Can you work these out from the model? Positions are in its coordinate system, mm. A direction names the side the tool comes from. Round coordinates to 2 decimals unless told otherwise and drop trailing zeros. Write each loop counter-clockwise with the first axis right and the second up, starting at its lowest first coordinate (ties: lowest second). Pieces come first, ordered by that corner, then holes. Notation, with made-up numbers: (-17, 21.25) -> (23, 21.25) arc R22 ccw to (23, 30.25) -> close; hole circle Ø10 at (-28.5, 31). An arc over 180 degrees is marked (long way). Write item = value, one per line. Start each with the question number.
1) If I drill on line 1 (Y direction, x = 0, z = 1.75); line 2 (Z direction, x = -7.5, y = 41.5); line 3 (X direction, y = 1, z = 1.5), over which ranges is the centre line in solid material (lowest first)?
2) Imagine slicing it at B-B, the plane y = 0. Please give me the cut outline in (x, z), then the cut area to 3 significant figures.
3) Imagine slicing it at D-D, the plane y = 16.5. Please give me the cut outline in (x, z), then the cut area to 3 significant figures.
4) I'm going to push flat-ended pins straight in: pin 1 (2.5 mm diameter, centred on x = -8.01, y = 37.25, fed in from -Z); pin 2 (2 mm diameter, centred on x = -2, y = 34, fed in from +Z); pin 3 (3 mm diameter, centred on x = -11, z = 1.5, fed in from +Y). Where does each tip first touch, or does it pass through?
5) Imagine slicing it at A-A, the plane x = 0. Please give me the cut outline in (y, z).
6) For faces 1 (the face through (-3.42, 3.13, 3.28)), 2 (the face through (-7.54, 36.35, 0.15)), which set-ups out of +Z, -Z, +X, -X, +Y, -Y let a thin tool reach every point of the face, with its end or its side?
7) Thinking about a two-plate mould opening in Y: for faces 3 (the face through (-10.27, 17.55, 0.78)), 4 (the face through (-2.217, -1.7, 3.131)), 5 (the face through (0, 43.598, 1)), 6 (the face through (7.793, 36.256, 0.15)), which applies, +Y half, -Y half, draft (parallel to the pull), parting line (faces both ways), or undercut?
8) Imagine slicing it at C-C, the plane z = 3.75. Please give me the cut outline in (x, y), then the cut area to 3 significant figures.
from build123d import *

# Parameters (mm, degrees)
F0_R     = 4.6355
F0_R_2   = 1.016
F1_DEPTH = 1.5748
F0_R_3   = 2.794
F2_DEPTH = 6.35
F3_SIZE  = 1.27


# Not quite as in the source:
# - a fillet or chamfer that OpenCascade refuses, or shapes differently, is made with other operations: its cross-section is extruded or revolved along the edge and cut away or added
# - a feature names something its author has since deleted; it is built from what else it names


with BuildPart() as f1:
    # F0 (on Top) → F1 (new body)
    with BuildSketch(Plane.XY):
        with BuildLine():
            Line((-14.2215059748, 35.912132599), (-6.2079540965, -1.3355919797))
            ThreePointArc((-6.2079540965, -1.3355919797), (0, -6.35), (6.2079540965, -1.3355919797))
            Line((6.2079540965, -1.3355919797), (14.2215059748, 35.912132599))
            ThreePointArc((14.2215059748, 35.912132599), (12.9533650869, 41.2378054632), (8.0135518783, 43.5977245787))
            Line((8.0135518783, 43.5977245787), (-8.0135518783, 43.5977245787))
            ThreePointArc((-8.0135518783, 43.5977245787), (-12.9533650869, 41.2378054632), (-14.2215059748, 35.912132599))
        make_face()
        Circle(F0_R, mode=Mode.SUBTRACT)
        with Locations((-8.0135518783, 37.2477245787)):
            Circle(F0_R_2, mode=Mode.SUBTRACT)
        with Locations((8.0135518783, 37.2477245787)):
            Circle(F0_R_2, mode=Mode.SUBTRACT)
    extrude(amount=F1_DEPTH)

    # F0 (on Top) → F2 (join)
    with BuildSketch(Plane.XY):
        Circle(F0_R)
        Circle(F0_R_3, mode=Mode.SUBTRACT)
    extrude(amount=F2_DEPTH)

    # F3
    f3_edges = [f1.edges().sort_by_distance(p)[0] for p in [
        (-9.029552, 37.247725, 1.5748),
        (6.997552, 37.247725, 1.5748),
    ]]
    chamfer(f3_edges, length=F3_SIZE)

    # F4: chamfer of 0.762 x 1.3198227154 on 1 edges, made by hand

    # F4_s1 → F4_t2 (revolve, cut)
    with BuildSketch(Plane.XZ):
        Polygon((4.6355, 5.0301772846), (3.8735, 6.35), (4.6355, 6.35), align=None)
    revolve(axis=Axis((0, 0, 6.35), (0, 0, 1)), mode=Mode.SUBTRACT)


solid = f1.part
Reported:
q1.line_1 = -4.64 to -2.79, 2.79 to 4.64
q1.line_2 = 0 to 1.57
q1.line_3 = -6.71 to -2.61, 2.61 to 6.71
q2.outline = (-6.5, 0) -> (-2.79, 0) -> (-2.79, 6.35) -> (-3.87, 6.35) -> (-4.64, 5.03) -> (-4.64, 1.57) -> (-6.5, 1.57) -> close; (2.79, 0) -> (6.5, 0) -> (6.5, 1.57) -> (4.64, 1.57) -> (4.64, 5.03) -> (3.87, 6.35) -> (2.79, 6.35) -> close
q2.area = 28.2 mm²
q3.outline = (-10.05, 0) -> (10.05, 0) -> (10.05, 1.57) -> (-10.05, 1.57) -> close
q3.area = 31.6 mm²
q4.pin_1 = 0
q4.pin_2 = 1.57
q4.pin_3 = 43.42
q5.outline = (-6.35, 0) -> (-2.79, 0) -> (-2.79, 6.35) -> (-3.87, 6.35) -> (-4.64, 5.03) -> (-4.64, 1.57) -> (-6.35, 1.57) -> close; (2.79, 0) -> (43.6, 0) -> (43.6, 1.57) -> (4.64, 1.57) -> (4.64, 5.03) -> (3.87, 6.35) -> (2.79, 6.35) -> close
q6.face_1 = +Z
q6.face_2 = +Z, -Z
q7.face_3 = -Y half
q7.face_4 = undercut
q7.face_5 = +Y half
q7.face_6 = undercut
q8.outline = circle Ø9.27 at (0, 0); hole circle Ø5.59 at (0, 0)
q8.area = 43.0 mm²
